```python
from build123d import *

# Parameters (mm, degrees)
EXTRUDE_1_DEPTH          = 6
PATTERN_CIRCULAR_1_COUNT = 23
SKETCH_3_R               = 17.5
SKETCH_3_R_2             = 4
CUT_EXTRUDE_1_DEPTH      = 7


with BuildPart() as part:
    # Эскиз2 → Бобышка-Вытянуть1 (new body)
    with BuildSketch(Plane.XY):
        with BuildLine():
            Line((0, 0), (0, 53.112541182))
            ThreePointArc((0, 53.112541182), (3.404315056, 54.38830771), (5.1317532, 57.587197939))
            ThreePointArc((5.1317532, 57.587197939), (5.93051423, 60.421485378), (7.471942626, 62.930509685))
            ThreePointArc((7.471942626, 62.930509685), (8.629226577, 62.782285913), (9.783585596, 62.612781672))
            ThreePointArc((9.783585596, 62.612781672), (10.590926988, 59.780926389), (10.595386193, 56.836238869))
            ThreePointArc((10.595386193, 56.836238869), (11.39571599, 53.289914934), (14.329592119, 51.142984079))
            Line((14.329592119, 51.142984079), (0, 0))
        make_face()
    extrude_1 = extrude(amount=EXTRUDE_1_DEPTH)

    # Круговой массив1: Бобышка-Вытянуть1 ×23 about axis
    pattern_circular_1_axis = Axis((0, 0, 0), (0, 0, 1))
    for i in range(1, PATTERN_CIRCULAR_1_COUNT):
        add(extrude_1.rotate(pattern_circular_1_axis, i * 360 / PATTERN_CIRCULAR_1_COUNT))

    # Эскиз3 → Вырез-Вытянуть1 (cut, through all)
    with BuildSketch(Plane.XY.offset(6)):
        Circle(SKETCH_3_R)
        with Locations((0, 30)):
            Circle(SKETCH_3_R_2)
        with Locations((25.980762114, 15)):
            Circle(SKETCH_3_R_2)
        with Locations((25.980762114, -15)):
            Circle(SKETCH_3_R_2)
        with Locations((0, -30)):
            Circle(SKETCH_3_R_2)
        with Locations((-25.980762114, -15)):
            Circle(SKETCH_3_R_2)
        with Locations((-25.980762114, 15)):
            Circle(SKETCH_3_R_2)
    extrude(amount=-CUT_EXTRUDE_1_DEPTH, mode=Mode.SUBTRACT)


solid = part.part
```
Input: part model. Units: mm. Frame: model coordinates. A direction names the side the tool comes from. Give positions to 0.01 mm unless a question says otherwise; leave off trailing zeros. Order: outer loops, then holes, each group sorted by start corner. A loop starts at its lowest first (then second) coordinate and runs counter-clockwise, first axis right, second up. Notation, with made-up numbers: M -5.5,62.25 L 7.5,62.25 A22 ccw 7.5,75.25 Z; hole C 26,-4 d1. An arc over 180 degrees is marked long. Return JSON: item names as keys, results as strings.
Item 1: Cut plane A-A (y = 15). Return loops of the section in (x, z), then the cut area to 3 significant figures.
Solutions:
{"outline": "M -52.95,0 L -29.98,0 L -29.98,6 L -52.95,6 Z; M -21.98,0 L -9.01,0 L -9.01,6 L -21.98,6 Z; M 9.01,0 L 21.98,0 L 21.98,6 L 9.01,6 Z; M 29.98,0 L 52.95,0 L 52.95,6 L 29.98,6 Z", "area": "431 mm^2"}
Item 2: First-contact query: P1, Ø1, axis at y = 39.5, z = 1.5, coming from the -X side. Flat tip, straight axial feed; report the tip coordinate or a pass-through.
Solutions:
{"P1": "x = -37.48"}
Item 3: Pull-direction query (Y, two-part tool) for faces 1 (the cylindrical face through (-14.081, -59.016, 2.958)), 2 (the cylindrical face through (21.986, 56.549, 2.958)), 3 (the cylindrical face through (59.8, -10, 3)); classes: +Y half, -Y half, draft (parallel to the pull), parting line (faces both ways), or undercut.
Solutions:
{"face 1": "-Y half", "face 2": "+Y half", "face 3": "undercut"}
Item 4: Access query for faces 4 (the cylindrical face through (-54.977, -25.85, 2.958)), 5 (the cylindrical face through (42.768, -43.146, 2.958)), 6 (the flat face through (-16, -9, 6)), 7 (the cylindrical face through (50.945, 33.096, 2.958)), 8 (the cylindrical face through (-5.947, 60.459, 2.958)). Directions: +Z, -Z, +X, -X, +Y, -Y. A direction counts if a zero-diameter tool reaches every point of the face in a straight line with its end or side. Return the directions, or none.
Solutions:
{"face 4": "+Z, -Z, -X", "face 5": "+Z, -Z, -Y", "face 6": "+Z, +X, -X, +Y, -Y", "face 7": "+Z, -Z, +X", "face 8": "+Z, -Z, +Y"}
Item 5: Ray query, probe 1 along Y at (x, z) = (-55.5, 4.25); probe 2 along Y at (x, z) = (27.5, 3.8); probe 3 along Y at (x, z) = (22.5, 5.6). Return the intervals inside material, ascending.
Solutions:
{"probe 1": "-30.2 to -26.38, -14.37 to -8.42, 0.47 to 6.92, 16.8 to 22.44", "probe 2": "-50.54 to -18.7, -11.3 to 11.3, 18.7 to 45.44", "probe 3": "-48.34 to -16.97, -13.03 to 13.03, 16.97 to 57.14"}
Item 6: Cut plane B-B (z = 2.8). State how many separate pieces and enclosed holes the cut face has, then the cut area to 3 significant figures.
Solutions:
{"separate pieces": "1", "enclosed holes": "7", "area": "8,970 mm^2"}
